Part model, mm, in its own coordinate system. Face numbers are marked on the shaded views. Give positions to 0.01 mm unless a question says otherwise; leave off trailing zeros. Write each loop counter-clockwise with the first axis right and the second up, starting at its lowest first coordinate (ties: lowest second). Pieces come first, ordered by that corner, then holes. Notation, with made-up numbers: M 87,84 L 113,84 A22 cw 113,116 Z; hole C 62.5,39.25 d2. An arc over 180 degrees is marked long. Use CSV: the item, a comma, the result in double quotes. Start each with the question number.
Item 1: Cut at B-B (z = -16). List the corners of the cut face in (x, y), then the cut area to 3 significant figures.
Item 2: Drill centre lines: line 1 (Y direction, x = 4.5, z = -6.5); line 2 (Y direction, x = 21.5, z = 15.5); line 3 (Z direction, x = 31.5, y = 15). Where is each one in solid material? Low to high. Write a range as [from, to].
Item 3: Mould opens along Z. For the marked faces 1, 2 and 3 say: released by +Z, released by -Z, zero draft, split by the parting line, or undercut.
Item 4: Cut at C-C (z = 8.5). Count the separate pieces of the cut face and the enclosed holes in it, then the cut area to 3 significant figures.
Item 5: Cut at A-A (y = 25.5). List the corners of the cut face in (x, z), then the cut area to 3 significant figures.
Item 6: Cut at D-D (z = 16.5). List the corners of the cut face in (x, y).
Item 7: Pin check, flat tips, straight feed: pin 1 (10 mm diameter, centred on x = 32, y = 31.5, fed in from +Z); pin 2 (12 mm diameter, centred on x = -25, y = 14.5, fed in from +Z); pin 3 (6 mm diameter, centred on x = -26, y = 23, fed in from +Z). Stop position of each tip, or through.
from build123d import *

# Parameters (mm, degrees)
EXTRUDE_1_DEPTH     = 52
EXTRUDE_2_DEPTH     = 1.5
SKETCH_4_R          = 11
CUT_EXTRUDE_1_DEPTH = 1.5


with BuildPart() as part:
    # 草图1 → 拉伸1 (new body)
    with BuildSketch(Plane(origin=(0, 0, 0), x_dir=(1, 0, 0), z_dir=(0, 1, 0))):
        with BuildLine():
            Line((-18.75, 20), (18.75, 20))
            ThreePointArc((18.75, 20), (38.75, 0), (18.75, -20))
            Line((18.75, -20), (-18.75, -20))
            ThreePointArc((-18.75, -20), (-38.75, 0), (-18.75, 20))
        make_face()
    extrude(amount=EXTRUDE_1_DEPTH)

    # 草图2 → 拉伸2 (add)
    with BuildSketch(Plane(origin=(0, 0, -20), x_dir=(-1, 0, 0), z_dir=(0, 0, -1))):
        Polygon((39, 74.5), (39, -22.5), (21.5, -22.5), (21.5, 0), (-21.5, 0), (-21.5, -22.5), (-39, -22.5), (-39, 74.5), (-21.5, 74.5), (-21.5, 52), (21.5, 52), (21.5, 74.5), align=None)
    extrude(amount=EXTRUDE_2_DEPTH)

    # 扫描4: sweep along a path in 草图3
    with BuildLine(Plane.XY) as sweep_4_path:
        Line((18.75, 51), (18.75, 5))
        ThreePointArc((18.75, 5), (14.356601718, -5.606601718), (3.75, -10))
        Line((3.75, -10), (-3.75, -10))
        ThreePointArc((-3.75, -10), (-14.356601718, -5.606601718), (-18.75, 5))
        Line((-18.75, 5), (-18.75, 51))
        ThreePointArc((-18.75, 51), (-14.356601718, 61.606601718), (-3.75, 66))
        Line((-3.75, 66), (3.75, 66))
        ThreePointArc((3.75, 66), (14.356601718, 61.606601718), (18.75, 51))
    # 草图4 → 扫描4 (sweep)
    with BuildSketch(Plane(origin=(0, 52, 0), x_dir=(-1, 0, 0), z_dir=(0, 1, 0))):
        with Locations((-18.75, 0)):
            Circle(SKETCH_4_R)
    sweep(path=sweep_4_path.line)

    # 草图6 → 切除-拉伸1 (cut)
    with BuildSketch(Plane(origin=(0, 0, -21.5), x_dir=(-1, 0, 0), z_dir=(0, 0, -1))):
        with BuildLine():
            Line((-32.5, 63), (-32.5, 59))
            ThreePointArc((-32.5, 59), (-30, 56.5), (-27.5, 59))
            Line((-27.5, 59), (-27.5, 63))
            ThreePointArc((-27.5, 63), (-30, 65.5), (-32.5, 63))
        make_face()
        with BuildLine():
            Line((32.5, 63), (32.5, 59))
            ThreePointArc((32.5, 59), (30, 56.5), (27.5, 59))
            Line((27.5, 59), (27.5, 63))
            ThreePointArc((27.5, 63), (30, 65.5), (32.5, 63))
        make_face()
        with BuildLine():
            Line((32.5, -11), (32.5, -7))
            ThreePointArc((32.5, -7), (30, -4.5), (27.5, -7))
            Line((27.5, -7), (27.5, -11))
            ThreePointArc((27.5, -11), (30, -13.5), (32.5, -11))
        make_face()
        with BuildLine():
            Line((-27.5, -11), (-27.5, -7))
            ThreePointArc((-27.5, -7), (-30, -4.5), (-32.5, -7))
            Line((-32.5, -7), (-32.5, -11))
            ThreePointArc((-32.5, -11), (-30, -13.5), (-27.5, -11))
        make_face()
    extrude(amount=-CUT_EXTRUDE_1_DEPTH, mode=Mode.SUBTRACT)


solid = part.part
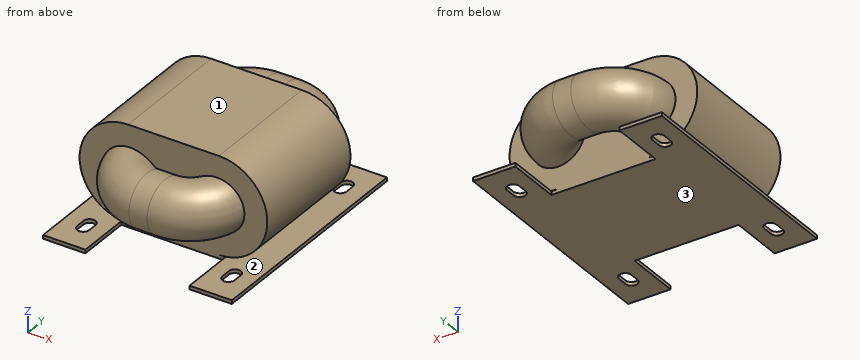
Worked answers:
1,outline,"M -30.75,0 L 30.75,0 L 30.75,52 L -30.75,52 Z"
1,area,"3,200 mm^2"
2,line 1,"y = [-18.88, -1.16], [0, 52], [57.16, 74.88]"
2,line 2,"y = [0, 52]"
2,line 3,"z = [-21.5, -20], [-15.41, 15.41]"
3,face 1,"released by +Z"
3,face 2,"undercut"
3,face 3,"released by -Z"
4,separate pieces,"1"
4,enclosed holes,"2"
4,area,"5,190 mm^2"
5,outline,"M -39,-21.5 L 39,-21.5 L 39,-20 L 18.75,-20 A20 ccw 18.75,20 L -18.75,20 A20 ccw -18.75,-20 L -39,-20 Z"
5,area,"2,870 mm^2"
6,outline,"M -30.05,0 L 30.05,0 L 30.05,52 L -30.05,52 Z"
7,pin 1,"stops at z = 18.22"
7,pin 2,"stops at z = 20"
7,pin 3,"stops at z = 19.54"
